```python
from build123d import *

# Parameters (mm, degrees)
SKETCH3_W                      = 243.3743418
SKETCH3_H                      = 19.05
BOSS_EXTRUDE1_DEPTH            = 1.905
F_6_CLEARANCE_HOLE1_AT_2_COUNT = 2
F_6_CLEARANCE_HOLE1_AT_2_PITCH = 224.3243418


with BuildPart() as part:
    # Sketch3 → Boss-Extrude1 (new body)
    with BuildSketch(Plane.XY):
        Rectangle(SKETCH3_W, SKETCH3_H)
    extrude(amount=BOSS_EXTRUDE1_DEPTH)

    # Sketch5 → #6 Clearance Hole1 (revolve, cut)
    with BuildSketch(Plane.YZ.offset(-112.1621709)):
        Polygon((0, 0), (0, 1.905), (2.15265, 1.905), (2.15265, 1.17475), (3.3274, 0), align=None)
    f_6_clearance_hole1 = revolve(axis=Axis((-112.1621709, 0, -6.35), (0, 0, 1)), mode=Mode.SUBTRACT)

    # #6 Clearance Hole1 at 2: #6 Clearance Hole1 ×2
    with Locations(*[(i * F_6_CLEARANCE_HOLE1_AT_2_PITCH, 0, 0) for i in range(1, F_6_CLEARANCE_HOLE1_AT_2_COUNT)]):
        add(f_6_clearance_hole1, mode=Mode.SUBTRACT)


solid = part.part
```
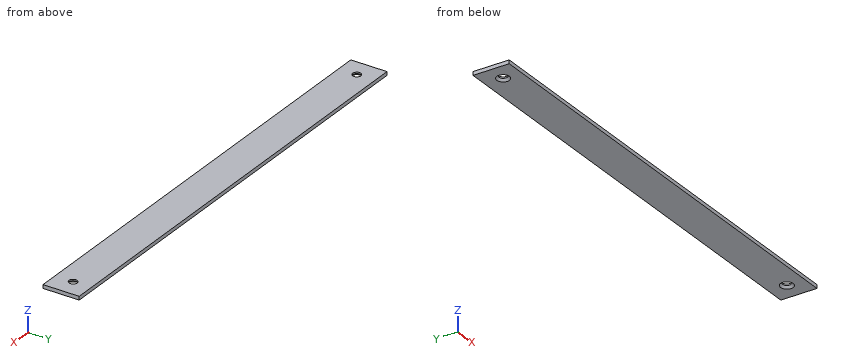
Input: part model. Units: mm. Frame: model coordinates. Coordinates: 2 decimals unless noted, no trailing zeros. Loops run counter-clockwise (first coordinate to the right, second up) from the corner with the lowest first, then second, coordinate; pieces in that order, holes last.
Q1. Section A-A, the plane y = 0. Return the cut outline in (x, z) (3 decimals).
Results are:
outline: (-121.687, 0) - (-115.49, 0) - (-114.315, 1.175) - (-114.315, 1.905) - (-121.687, 1.905) - close; (-110.01, 1.175) - (-108.835, 0) - (108.835, 0) - (110.01, 1.175) - (110.01, 1.905) - (-110.01, 1.905) - close; (114.315, 1.175) - (115.49, 0) - (121.687, 0) - (121.687, 1.905) - (114.315, 1.905) - close
Q2. Contact query for a flat-ended pin moving along its axis: pin 1 (5.5 mm diameter, centred on x = -112.16, y = 0, fed in from -Z). Output: stop coordinate, or through.
Results are:
pin 1: stops at z = 0.58
Q3. Line query: line 1 along X through (y, z) = (0, 1.3); line 2 along Y through (x, z) = (-111, 1) (3 decimals); line 3 along X through (y, z) = (0, 1.1). Output: solid intervals per line, ascending.
Results are:
line 1: x = -121.69 to -114.31, -110.01 to 110.01, 114.31 to 121.69
line 2: y = -9.525 to -2.016, 2.016 to 9.525
line 3: x = -121.69 to -114.39, -109.93 to 109.93, 114.39 to 121.69
